For this review, use the dimensioned drawing (mm, ordinates from the lowest corner) and the shaded views. A direction names the side the tool comes from. Coordinates: 2 decimals unless noted, no trailing zeros. Order: outer loops, then holes, each group sorted by start corner. A loop starts at its lowest first (then second) coordinate and runs counter-clockwise, first axis right, second up. Notation, with made-up numbers: M -22.5,87.5 L 21.5,87.5 A9 cw 21.5,103.5 Z; hole C 83,26 d10. An arc over 180 degrees is marked long. Answer in a Markdown table with one row per item.
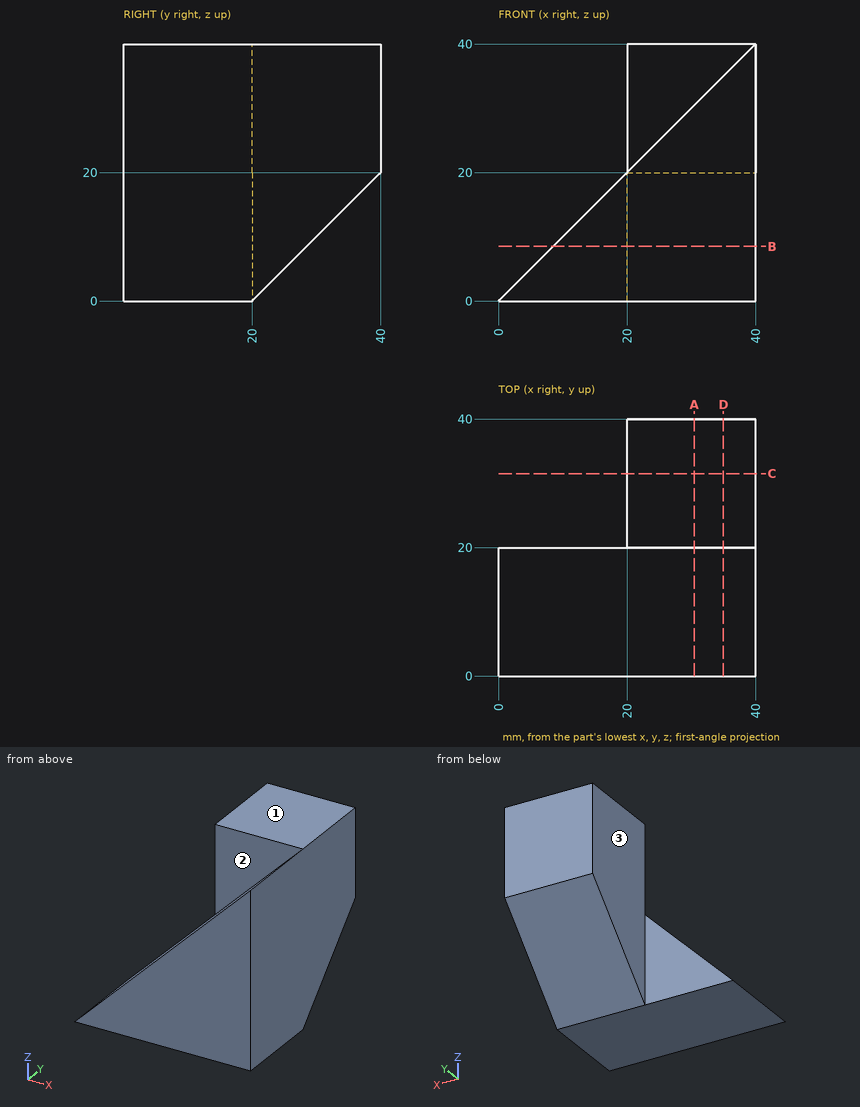
(1) To check wall thickness, follow line 1 (X direction, y = 29, z = 10); line 2 (Y direction, x = 7.5, z = 5.5); line 3 (Y direction, x = 24, z = 17.5). State the ranges of each line that lie inside material, in increasing order. Write a range as [from, to].
Report:
| item | result |
|---|---|
| line 1 | [20, 40] |
| line 2 | [0, 20] |
| line 3 | [0, 37.5] |
(2) Take a section at C-C (y = 31.5). Write out the cut boundary in (x, z), then the cut area to 3 significant figures.
Report:
| item | result |
|---|---|
| outline | M 20,11.5 L 40,11.5 L 40,40 L 20,40 Z |
| area | 570 mm^2 |
(3) Insertion check: P1, Ø4, axis at x = 14, z = 5.5, coming from the +Y side; P2, Ø6, axis at y = 32.5, z = 14, coming from the -X side; P3, Ø3, axis at x = 21.5, y = 23.5, coming from the -Z side. Each pin has a flat end and moves straight along its axis. Give the tip position at first contact, or say it passes through.
Report:
| item | result |
|---|---|
| P1 | y = 20 |
| P2 | x = 20 |
| P3 | z = 2 |
(4) Take a section at D-D (x = 35). Write out the cut boundary in (y, z).
Report:
| item | result |
|---|---|
| outline | M 0,0 L 20,0 L 40,20 L 40,40 L 20,40 L 20,35 L 0,35 Z |
(5) Take a section at B-B (z = 8.5). Write out the cut boundary in (x, y), then the cut area to 3 significant figures.
Report:
| item | result |
|---|---|
| outline | M 8.5,0 L 40,0 L 40,28.5 L 20,28.5 L 20,20 L 8.5,20 Z |
| area | 800 mm^2 |
(6) Machinability: for the marked faces 1, 2 and 3, which of the approach directions +Z, -Z, +X, -X, +Y, -Y give a long, thin tool a straight path to every point of the face, cutting with its end or side? Answer none if there is none.
Report:
| item | result |
|---|---|
| face 1 | +Z, +X, -X, +Y, -Y |
| face 2 | +Z, -X, -Y |
| face 3 | +Z, -Z, -X, +Y |
(7) Take a section at A-A (x = 30.5). Write out the cut boundary in (y, z).
Report:
| item | result |
|---|---|
| outline | M 0,0 L 20,0 L 40,20 L 40,40 L 20,40 L 20,30.5 L 0,30.5 Z |
